from build123d import *

# Parameters (mm, degrees)
SKETCH2_W           = 139.7
SKETCH2_H           = 139.7
SKETCH2_R           = 63.5
BOSS_EXTRUDE2_DEPTH = 6.35
SKETCH2_4_W         = 6.35
SKETCH2_4_H         = 38.1
SKETCH2_4_W_2       = 38.1
SKETCH2_4_H_2       = 6.35
BOSS_EXTRUDE3_DEPTH = 6.35


with BuildPart() as part:
    # Sketch2 → Boss-Extrude2 (new body)
    with BuildSketch(Plane(origin=(0, 0, 0), x_dir=(1, 0, 0), z_dir=(0, 1, 0))):
        Rectangle(SKETCH2_W, SKETCH2_H)
        with Locations(Location((0, 0, 0), (0, 0, 270))):
            Circle(SKETCH2_R, mode=Mode.SUBTRACT)
    extrude(amount=BOSS_EXTRUDE2_DEPTH)

    # Sketch2_4 → Boss-Extrude3 (add)
    with BuildSketch(Plane(origin=(0, 0, 0), x_dir=(1, 0, 0), z_dir=(0, 1, 0))):
        with Locations((-73.025, 0)):
            Rectangle(SKETCH2_4_W, SKETCH2_4_H)
        with Locations((0, -73.025)):
            Rectangle(SKETCH2_4_W_2, SKETCH2_4_H_2)
        with Locations((73.025, 0)):
            Rectangle(SKETCH2_4_W, SKETCH2_4_H)
        with Locations((0, 73.025)):
            Rectangle(SKETCH2_4_W_2, SKETCH2_4_H_2)
    extrude(amount=BOSS_EXTRUDE3_DEPTH)


solid = part.part
Verification items for the finished model (mm, model axes). A direction names the side the tool comes from. Coordinates: 2 decimals unless noted, no trailing zeros. Loops run counter-clockwise (first coordinate to the right, second up) from the corner with the lowest first, then second, coordinate; pieces in that order, holes last. Notation, with made-up numbers: M 45.5,-30 L 55.5,-30 A12 cw 55.5,-26 Z; hole C -40,29 d5. An arc over 180 degrees is marked long. One line per item, written item: value.
1. Set-up check for faces 1 (the flat face through (-73, 3, 19.05)), 2 (the flat face through (19.05, 3, -73)), 3 (the flat face through (44, 3, 69.85)), 4 (the flat face through (-45, 3, -69.85)): record each of +Z, -Z, +X, -X, +Y, -Y from which the full face is reachable in a straight line by a thin tool's end or side.
Answers follow:
face 1: +Z, -X, +Y, -Y
face 2: -Z, +X, +Y, -Y
face 3: +Z, +X, +Y, -Y
face 4: -Z, -X, +Y, -Y
2. Section check B-B on z = 0. Record the cut outline in (x, y), plus the area to 3 significant figures.
Answers follow:
outline: M -76.2,0 L -63.5,0 L -63.5,6.35 L -76.2,6.35 Z; M 63.5,0 L 76.2,0 L 76.2,6.35 L 63.5,6.35 Z
area: 161 mm^2
3. Section check A-A on y = 3. Record the cut outline in (x, z).
Answers follow:
outline: M -76.2,-19.05 L -69.85,-19.05 L -69.85,-69.85 L -19.05,-69.85 L -19.05,-76.2 L 19.05,-76.2 L 19.05,-69.85 L 69.85,-69.85 L 69.85,-19.05 L 76.2,-19.05 L 76.2,19.05 L 69.85,19.05 L 69.85,69.85 L 19.05,69.85 L 19.05,76.2 L -19.05,76.2 L -19.05,69.85 L -69.85,69.85 L -69.85,19.05 L -76.2,19.05 Z; hole C 0,0 d127
4. Mould release check, pull along X, two halves, no side actions. Record for faces 5 (the flat face through (-19.05, 3, 73)), 6 (the cylindrical face through (-61.99, 3.13, -13.77)), 7 (the flat face through (19.05, 3, 73)), 8 (the flat face through (44, 3, -69.85)): pulls with the +X half, pulls with the -X half, needs draft (parallel to the pull), parting line crosses it, or undercut.
Answers follow:
face 5: pulls with the -X half
face 6: undercut
face 7: pulls with the +X half
face 8: needs draft
5. Section check C-C on x = 0. Record the cut outline in (y, z), plus the area to 3 significant figures.
Answers follow:
outline: M 0,-76.2 L 6.35,-76.2 L 6.35,-63.5 L 0,-63.5 Z; M 0,63.5 L 6.35,63.5 L 6.35,76.2 L 0,76.2 Z
area: 161 mm^2
6. Gauge pin test, flat ends, axial feed: P1, Ø3, axis at y = 1, z = 36.5, coming from the -X side; P2, Ø1.9, axis at x = 73, y = 4.5, coming from the +Z side; P3, Ø3, axis at y = 3, z = 72, coming from the +X side. Record the tip position at first contact, or that the pin passes through.
Answers follow:
P1: x = -69.85
P2: z = 19.05
P3: x = 19.05
7. Material ranges on line 1 along X through (y, z) = (2, 0); line 2 along X through (y, z) = (1.5, -68.5); line 3 along Z through (x, y) = (44, 5), recorded low to high. Write a range as from..to.
Answers follow:
line 1: -76.2..-63.5, 63.5..76.2
line 2: -69.85..69.85
line 3: -69.85..-45.78, 45.78..69.85
